Autodesk Inventor part; units mm, degrees
ref_plane "Work Plane1" through (33.575, 0, 0) normal (0, 0, -1) x (1, 0, 0)
ref_plane "YZ Plane" through (0, 0, 0) normal (1, 0, 0) x (0, 1, 0)
ref_plane "XZ Plane" through (0, 0, 0) normal (0, 1, 0) x (-1, 0, 0)
sketch "Esquisse1" plane through (0, 0, 0) normal (0, 0, 1) x (1, 0, 0)
  line L0 (0, 0) -> (8, 0)
  line L1 (8, 0) -> (8, 1.5)
  line L2 (8, 1.5) -> (2.65, 1.5)
  line L3 (2.65, 1.5) -> (2.3433, 1.5)
  line L4 (2.3433, 1.5) -> (1.65, 1.5)
  line L5 (1.65, 1.5) -> (0.35, 2.8)
  line L6 (0.35, 2.8) -> (0, 2.8)
  line L7 (0, 2.8) -> (0, 0)
  line L8 (2.65, 1.5) -> (1.65, 1.5) construction
  line L9 (-1.6, 0) -> (9.6, 0)
  line L10 (0, 3.36) -> (0, -0.56)
  dimension "d0" = 8
  dimension "d1" = 45
  dimension "d2" = 0.3067
  dimension "d3" = 5.35
  dimension "d4" = 1.65
  dimension "d5" = 3
  dimension "d6" = 3
  dimension "d7" = 5.6
revolve "Corps" add sketch "Esquisse1" angle 360 about axis through (0, 0, 0) along (1, 0, 0)
sketch "Esquisse2" plane through (0, 0, 0) normal (-1, 0, 0) x (0, 0, 1)
  line L0 (2.8, -0.4) -> (-2.8, -0.4)
  line L1 (-2.8, -0.4) -> (-2.8, 0.4)
  line L2 (-2.8, 0.4) -> (2.8, 0.4)
  line L3 (2.8, 0.4) -> (2.8, -0.4)
  line L4 (0, 0.4) -> (0, -0.4) construction
  line L5 (-2.8, 0) -> (2.8, 0) construction
  line L6 (0, 2.8) -> (0, 0)
  dimension "d15" = 0.8
  dimension "d16" = 5.6
extrude "Rainure" cut sketch "Esquisse2" against normal blind 0.85
thread "Filetage"
chamfer "Chanfrein1" distance 0.3067 distance2 0.1534 1 edges at (8, -1.5, 0) measured on face at (8, 0.263, 0.1197)
ref_plane "Work Plane1" through (33.575, 0, 0) normal (0, 0, -1) x (1, 0, 0)
equation "\"d0\" = NLG"
equation "\"d1\" = 0.5 * SEWI"
equation "\"d2\" = GAL"
equation "\"d3\" = GEL"
equation "\"d4\" = KOH"
equation "\"d5\" = BDM"
equation "\"d6\" = GD"
equation "\"d7\" = KOD"
equation "\"d15\" = SBR"
equation "\"d16\" = KOD"
equation "\"d8\" = STI"
equation "\"d10\" = GEL"
equation "\"d12\" = -0.5 * SPD + 0.5 * GD"
equation "\"d13\" = 0.5 * GAL"
equation "\"NLG\" = 8"
equation "\"GAL\" = 0.61345 * PTC"
equation "\"GEL\" = 5.35"
equation "\"KOH\" = 1.65"
equation "\"KOD\" = 5.6"
equation "\"SEWI\" = 90deg"
equation "\"BDM\" = NND"
equation "\"GD\" = NND"
equation "\"SBR\" = 0.8"
equation "\"STI\" = 0.85"
equation "\"SPD\" = NND - 1.2269 * PTC"
equation "\"GUL\" = 0.61345 * PTC"
equation "\"PTC\" = 0.5"
equation "\"EPV\" = 3.15"
equation "\"THREADDIA\" = 3"
equation "\"TOA\" = 30deg"
equation "\"NND\" = 3"
equation "\"GD1\" = THREADDIA - 1.2269 * PTC"
properties part number "DIN 963 - M3 x 8" material "Acier, doux"
Design review of the part built by this model. Coordinates are the model's own, in mm. A direction names the side the tool comes from. Give positions to 0.01 mm unless a question says otherwise; leave off trailing zeros. Loops run counter-clockwise (first coordinate to the right, second up) from the corner with the lowest first, then second, coordinate; pieces in that order, holes last. Notation, with made-up numbers: M -38.5,-20 L -0.5,-20 A13 ccw -0.5,-3 Z; hole C -19,-31.5 d4. An arc over 180 degrees is marked long. Return JSON: item names as keys, results as strings. Group by question number.
Item 1: Mouldability with a two-part tool opening along Y and no side actions: class faces 1 (the flat face through (0.4, 0.4, 0)), 2 (the flat face through (0.85, 0, 0)), 3 (the flat face through (0, 1, 0)), 4 (the cylindrical face through (4.7, -1.5, -0.07)) as released by +Y, released by -Y, zero draft, split by the parting line, or undercut.
Item 2: Insertion check: pin 1 Ø1.5 at (x, z) = (7, -1.5) entering from +Y; pin 2 Ø1.5 at (y, z) = (1.5, -0.5) entering from +X; pin 3 Ø0.6 at (y, z) = (0, 0) entering from -X. Each pin has a flat end and moves straight along its axis. Give the tip position at first contact, or say it passes through.
Item 3: We need section A-A (y = 0). Give the boundary of the cut face in (x, z).
Item 4: We need section D-D (x = 0.75). Give the boundary of the cut face in (y, z), and give its area (3 significant figures).
Item 5: Tool access review of faces 5 (the flat face through (0.4, -0.4, 0)), 6 (the flat face through (8, 0, 0)): name each direction out of +Z, -Z, +X, -X, +Y, -Y from which nothing blocks a thin tool from reaching the whole face with its end or side.
Item 6: We need section C-C (x = 5.5). Give the boundary of the cut face in (y, z).
Item 7: We need section B-B (z = 0). Give the boundary of the cut face in (x, y).
Item 8: For probe 1 along Z at (x, y) = (2.5, -0.9); probe 2 along Z at (x, y) = (2.25, 0.3); probe 3 along Y at (x, z) = (0.75, -1.6), list the stretches that pass through material, from the lowest coordinate up.
Output:
{
 "1": {"face 1": "undercut", "face 2": "undercut", "face 3": "zero draft", "face 4": "split by the parting line"},
 "2": {"pin 1": "stops at y = 1.3", "pin 2": "stops at x = 8", "pin 3": "stops at x = 0.85"},
 "3": {"outline": "M 0.85,-2.3 L 1.65,-1.5 L 7.85,-1.5 L 8,-1.19 L 8,1.19 L 7.85,1.5 L 1.65,1.5 L 0.85,2.3 Z"},
 "4": {"outline": "M -0.4,-2.37 L -0.4,2.37 A2.4 ccw Z; M 0.4,-2.37 A2.4 ccw 0.4,2.37 Z", "area": "14.3 mm^2"},
 "5": {"face 5": "+Z, -Z, -X", "face 6": "+Z, -Z, +X, +Y, -Y"},
 "6": {"outline": "C 0,0 d3"},
 "7": {"outline": "M 0,-2.8 L 0.35,-2.8 L 1.65,-1.5 L 7.85,-1.5 L 8,-1.19 L 8,1.19 L 7.85,1.5 L 1.65,1.5 L 0.35,2.8 L 0,2.8 L 0,0.4 L 0.85,0.4 L 0.85,-0.4 L 0,-0.4 Z"},
 "8": {"probe 1": "z = -1.2 to 1.2", "probe 2": "z = -1.47 to 1.47", "probe 3": "y = -1.79 to -0.4, 0.4 to 1.79"}
}
